The model under review builds one solid part; all positions refer to its coordinate system, in mm. A direction names the side the tool comes from. Give positions to 0.01 mm unless a question says otherwise; leave off trailing zeros. Loops run counter-clockwise (first coordinate to the right, second up) from the corner with the lowest first, then second, coordinate; pieces in that order, holes last. Notation, with made-up numbers: (81.5, 84.5) - (97.5, 84.5) arc R32 cw to (97.5, 120.5) - close; hole circle Ø2 at (13, 81.5). An arc over 180 degrees is marked (long way). Return JSON: item names as keys, results as strings. Group by question number.
from build123d import *

# Parameters (mm, degrees)
SALIENTE_EXTRUIR1_DEPTH = 100
CROQUIS2_R              = 4
CORTAR_EXTRUIR1_DEPTH   = 23
CORTAR_EXTRUIR3_DEPTH   = 101


with BuildPart() as part:
    # Croquis1 → Saliente-Extruir1 (new body)
    with BuildSketch(Plane(origin=(0, 0, 0), x_dir=(0, 0, -1), z_dir=(1, 0, 0))):
        with BuildLine():
            Line((0, 0), (-22.597979746, 0))
            ThreePointArc((-22.597979746, 0), (-23.363346611, 0.152240935), (-24.012193309, 0.585786438))
            Line((-24.012193309, 0.585786438), (-34.121320344, 10.694913472))
            ThreePointArc((-34.121320344, 10.694913472), (-34.771638598, 13.964284113), (-32, 15.816233816))
            Line((-32, 15.816233816), (-27, 15.816233816))
            ThreePointArc((-27, 15.816233816), (-25.585786438, 16.402020254), (-25, 17.816233816))
            Line((-25, 17.816233816), (-25, 27.816233816))
            ThreePointArc((-25, 27.816233816), (-25.152240935, 28.581600681), (-25.585786438, 29.230447378))
            Line((-25.585786438, 29.230447378), (-37.656854249, 41.30151519))
            ThreePointArc((-37.656854249, 41.30151519), (-39.39103626, 50.019836899), (-32, 54.95836944))
            Line((-32, 54.95836944), (-24, 54.95836944))
            ThreePointArc((-24, 54.95836944), (-22.585786438, 55.544155877), (-22, 56.95836944))
            Line((-22, 56.95836944), (-22, 69.95836944))
            ThreePointArc((-22, 69.95836944), (-22.152240935, 70.723736304), (-22.585786438, 71.372583002))
            Line((-22.585786438, 71.372583002), (-35.606601718, 84.393398282))
            ThreePointArc((-35.606601718, 84.393398282), (-38.858192988, 100.740251485), (-25, 110))
            Line((-25, 110), (0, 110))
            Line((0, 110), (0, 0))
        make_face()
    extrude(amount=SALIENTE_EXTRUIR1_DEPTH)

    # Croquis2 → Cortar-Extruir1 (cut, through all)
    with BuildSketch(Plane.XY.offset(22)):
        with Locations((10, 63.45836944)):
            Circle(CROQUIS2_R)
        with Locations((90, 63.45836944)):
            Circle(CROQUIS2_R)
    extrude(amount=-CORTAR_EXTRUIR1_DEPTH, mode=Mode.SUBTRACT)

    # Croquis3 → Cortar-Extruir3 (cut, through all)
    with BuildSketch(Plane(origin=(100, 0, 0), x_dir=(0, 0, -1), z_dir=(1, 0, 0))):
        with BuildLine():
            Line((-24, 52.95836944), (-32, 52.95836944))
            ThreePointArc((-32, 52.95836944), (-37.543277195, 49.254470034), (-36.242640687, 42.715728753))
            Line((-36.242640687, 42.715728753), (-24.171572875, 30.644660941))
            ThreePointArc((-24.171572875, 30.644660941), (-23.30448187, 29.346967545), (-23, 27.816233816))
            Line((-23, 27.816233816), (-23, 17.816233816))
            ThreePointArc((-23, 17.816233816), (-24.171572875, 14.987806691), (-27, 13.816233816))
            Line((-27, 13.816233816), (-32, 13.816233816))
            ThreePointArc((-32, 13.816233816), (-32.923879533, 13.198917248), (-32.707106781, 12.109127035))
            Line((-32.707106781, 12.109127035), (-22.597979746, 2))
            Line((-22.597979746, 2), (-2, 2))
            Line((-2, 2), (-2, 108))
            Line((-2, 108), (-25, 108))
            ThreePointArc((-25, 108), (-37.010433923, 99.974884621), (-34.192388155, 85.807611845))
            Line((-34.192388155, 85.807611845), (-21.171572875, 72.786796564))
            ThreePointArc((-21.171572875, 72.786796564), (-20.30448187, 71.489103169), (-20, 69.95836944))
            Line((-20, 69.95836944), (-20, 56.95836944))
            ThreePointArc((-20, 56.95836944), (-21.171572875, 54.129942315), (-24, 52.95836944))
        make_face()
    extrude(amount=-CORTAR_EXTRUIR3_DEPTH, mode=Mode.SUBTRACT)


solid = part.part
Item 1: For L1, parallel to Y at x = 10, z = 0.95; L2, parallel to Y at x = 13.5, z = 12; L3, parallel to Y at x = 50, z = 27.5, list the stretches that pass through material, from the lowest coordinate up. Write a range as from..to.
Item 2: Take a section at C-C (z = 29.5). State the section outline as (x, y) points, then the cut area to 3 significant figures.
Item 3: For P1, Ø4, axis at y = 18, z = 34.5, coming from the -X side; P2, Ø1.5, axis at x = 52, z = 30.5, coming from the +Y side; P3, Ø9, axis at x = 10, y = 63.46, coming from the +Z side; P4, Ø2.5, axis at x = 44.5, z = 29, coming from the -Y side, all flat-tipped, find the tip position at first contact; note any pin that passes through.
Item 4: Mouldability with a two-part tool opening along X and no side actions: class faces 1 (the face through (100, 63, 21)), 2 (the face through (50.7, 36.765, 30.292)), 3 (the face through (7.05, 66.16, 21.01)) as +X half, -X half, draft (parallel to the pull), parting line (faces both ways), or undercut.
Item 5: Take a section at B-B (y = 102.5). State the section outline as (x, z) points.
Item 6: Take a section at A-A (z = 5). State the section outline as (x, y) points, then the cut area to 3 significant figures.
Item 7: Tool access review of faces 4 (the face through (49, 23, 25)), 5 (the face through (50.7, 29.367, 23.313)), 6 (the face through (49.3, 5.57, 28.996)): name each direction out of +Z, -Z, +X, -X, +Y, -Y from which nothing blocks a thin tool from reaching the whole face with its end or side.
Check sheet entries:
{
 "1": {"L1": "y = 0..59.46, 67.46..110", "L2": "y = 0..2, 108..110", "L3": "y = 4.07..6.9, 13.82..15.82, 31.14..33.97, 52.96..54.96, 76.29..79.12, 107.76..109.79"},
 "2": {"outline": "(0, 6.07) - (100, 6.07) - (100, 8.9) - (0, 8.9) - close; (0, 13.82) - (100, 13.82) - (100, 15.82) - (0, 15.82) - close; (0, 33.14) - (100, 33.14) - (100, 35.97) - (0, 35.97) - close; (0, 52.96) - (100, 52.96) - (100, 54.96) - (0, 54.96) - close; (0, 78.29) - (100, 78.29) - (100, 81.12) - (0, 81.12) - close; (0, 107.2) - (100, 107.2) - (100, 109.31) - (0, 109.31) - close", "area": "1,460 mm^2"},
 "3": {"P1": "passes through", "P2": "stops at y = 109.23", "P3": "stops at z = 22", "P4": "stops at y = 4.32"},
 "4": {"face 1": "+X half", "face 2": "draft", "face 3": "undercut"},
 "5": {"outline": "(0, 0) - (100, 0) - (100, 2) - (0, 2) - close; (0, 35.62) - (100, 35.62) - (100, 37.99) - (0, 37.99) - close"},
 "6": {"outline": "(0, 0) - (100, 0) - (100, 2) - (0, 2) - close; (0, 108) - (100, 108) - (100, 110) - (0, 110) - close", "area": "400 mm^2"},
 "7": {"face 4": "+Z, +X, -X", "face 5": "+X, -X", "face 6": "+Z, +X, -X, -Y"}
}
